For this review, take the finished solid that the model builds, in its own axes (mm). Coordinates: 2 decimals unless noted, no trailing zeros. Write each loop counter-clockwise with the first axis right and the second up, starting at its lowest first coordinate (ties: lowest second). Pieces come first, ordered by that corner, then holes.
```python
from build123d import *

# Parameters (mm, degrees)
SWEEP1_PROFILE_R = 2.5


with BuildPart() as part:
    # Sweep1: sweep along a curve in space
    with BuildLine() as sweep1_path:
        Line((0, 0, 0), (0, 30, 0))
        Line((0, 30, 0), (0, 73.301270189, -25))
        Line((0, 73.301270189, -25), (20, 73.301270189, -25))
        Line((20, 73.301270189, -25), (20, 112.70180787, -55.783073766))
        Line((20, 112.70180787, -55.783073766), (20, 103.46688574, -67.60323507))
        Line((20, 103.46688574, -67.60323507), (20, 188.337375311, -116.60323507))
        Line((20, 188.337375311, -116.60323507), (20, 196.337375311, -102.74682861))
        Line((20, 196.337375311, -102.74682861), (3.978461048, 196.337375311, -102.74682861))
    # Sweep1 profile (on start of the path) → Sweep1 (sweep)
    with BuildSketch(Plane.ZX):
        Circle(SWEEP1_PROFILE_R)
    sweep(path=sweep1_path.line, transition=Transition.RIGHT)


solid = part.part
```
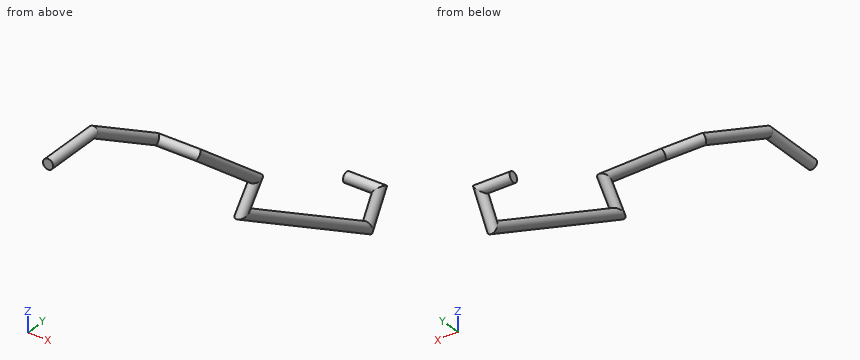
Q1. For probe 1 along Z at (x, y) = (19.25, 107.5); probe 2 along Y at (x, z) = (5, -101); probe 3 along Z at (x, y) = (-1.5, 71), list the stretches that pass through material, from the lowest coordinate up.
Ans:
probe 1: z = -72.69 to -67.18, -66.31 to -58.57, -54.75 to -48.69
probe 2: y = 194.55 to 198.13
probe 3: z = -25.98 to -21.36
Q2. Add section A-A (x = 7.5). State the section outline as (y, z) points.
Ans:
outline: circle Ø5 at (73.3, -25); circle Ø5 at (196.34, -102.75)
Q3. Clearance check with flat-ended pins moving along their axes: pin 1 Ø6 at (x, z) = (18, -17) entering from +Y; pin 2 Ø3 at (x, z) = (12.5, -100.5) entering from -Y; pin 3 Ø8 at (x, y) = (1.5, 24) entering from -Z; pin 4 Ø2.5 at (y, z) = (197, -103.5) entering from -X. State where each tip first meets the part, or that it passes through.
Ans:
pin 1: passes through
pin 2: stops at y = 193.95
pin 3: stops at z = -2.5
pin 4: stops at x = 3.98
